Geometry check sheet. Reference: the model listing, model coordinates, mm. A direction names the side the tool comes from. Round coordinates to 2 decimals unless told otherwise and drop trailing zeros. Order: outer loops, then holes, each group sorted by start corner. A loop starts at its lowest first (then second) coordinate and runs counter-clockwise, first axis right, second up. Notation, with made-up numbers: M 81.25,-19 L 129.25,-19 A15 cw 129.25,-2 Z; hole C 65.5,6 d5. An arc over 180 degrees is marked long. Return JSON: item names as keys, results as strings. Group by question number.
```python
from build123d import *

# Parameters (mm, degrees)
F1_R     = 300
F1_R_2   = 275
F2_DEPTH = 25
F3_W     = 25
F3_H     = 25
F4_DEPTH = 410
F6_R     = 300
F6_R_2   = 275
F7_DEPTH = 25


with BuildPart() as f2:
    # F1 (on face) → F2 (new body)
    with BuildSketch(Plane.XY):
        Circle(F1_R)
        Circle(F1_R_2, mode=Mode.SUBTRACT)
    extrude(amount=F2_DEPTH)

    # F3 (on face) → F4 (join)
    with BuildSketch(Plane.XY.offset(25)):
        with Locations((0, 287.215762)):
            Rectangle(F3_W, F3_H)
        with Locations((-287.215762, 0)):
            Rectangle(F3_W, F3_H)
        with Locations((0, -287.215762)):
            Rectangle(F3_W, F3_H)
        with Locations((287.215762, 0)):
            Rectangle(F3_W, F3_H)
    extrude(amount=F4_DEPTH)

    # F6 (on offset) → F7 (join)
    with BuildSketch(Plane.XY.offset(435)):
        Circle(F6_R)
        Circle(F6_R_2, mode=Mode.SUBTRACT)
    extrude(amount=F7_DEPTH)


solid = f2.part
```
Q1. Depth check by flat-ended pin: pin 1 Ø7.5 at (y, z) = (-283.5, 160.5) entering from -X; pin 2 Ø20 at (x, z) = (-4, 245.5) entering from -Y; pin 3 Ø20 at (y, z) = (286.5, 318) entering from +X. Enter the tip coordinate at first touch or a pass-through.
Q2. Section check B-B on z = 268. Record the cut outline in (x, y), plus the area to 3 significant figures.
Q3. Release check for a two-part mould opening along X. For faces 1 (the face through (-39.054, 297.447, 447.325)), 2 (the face through (274.716, 0, 227)), 3 (the face through (132, -243, 435)) record: +X half, -X half, draft (parallel to the pull), parting line (faces both ways), or undercut.
Q4. Set-up check for faces 4 (the face through (287, 12.5, 227)), 5 (the face through (12.5, -287, 227)), 6 (the face through (0, -274.716, 227)), 7 (the face through (287, -12.5, 227)): record each of +Z, -Z, +X, -X, +Y, -Y from which the full face is reachable in a straight line by a thin tool's end or side.
Q5. Material ranges on line 1 along Z through (x, y) = (-217, -189.5); line 2 along Y through (x, z) = (-6.5, 208.5); line 3 along Y through (x, z) = (0, 443), recorded low to high.
Q6. Section check D-D on x = 200.5. Record the cut outline in (y, z), plus the area to 3 significant figures.
Q7. Section check A-A on x = 0. Record the cut outline in (y, z), plus the area to 3 significant figures.
Geometry check:
{
 "1": {"pin 1": "stops at x = -12.5", "pin 2": "stops at y = -299.72", "pin 3": "stops at x = 12.5"},
 "2": {"outline": "M -299.72,-12.5 L -274.72,-12.5 L -274.72,12.5 L -299.72,12.5 Z; M -12.5,-299.72 L 12.5,-299.72 L 12.5,-274.72 L -12.5,-274.72 Z; M -12.5,274.72 L 12.5,274.72 L 12.5,299.72 L -12.5,299.72 Z; M 274.72,-12.5 L 299.72,-12.5 L 299.72,12.5 L 274.72,12.5 Z", "area": "2,500 mm^2"},
 "3": {"face 1": "parting line", "face 2": "undercut", "face 3": "draft"},
 "4": {"face 4": "+X, -X, +Y", "face 5": "+X, +Y, -Y", "face 6": "+Z, -Z, +X, -X", "face 7": "+X, -X, -Y"},
 "5": {"line 1": "z = 0 to 25, 435 to 460", "line 2": "y = -299.72 to -274.72, 274.72 to 299.72", "line 3": "y = -300 to -275, 275 to 300"},
 "6": {"outline": "M -223.16,0 L -188.21,0 L -188.21,25 L -223.16,25 Z; M -223.16,435 L -188.21,435 L -188.21,460 L -223.16,460 Z; M 188.21,0 L 223.16,0 L 223.16,25 L 188.21,25 Z; M 188.21,435 L 223.16,435 L 223.16,460 L 188.21,460 Z", "area": "3,490 mm^2"},
 "7": {"outline": "M -300,0 L -275,0 L -275,25 L -274.72,25 L -274.72,435 L -275,435 L -275,460 L -300,460 L -300,435 L -299.72,435 L -299.72,25 L -300,25 Z; M 274.72,25 L 275,25 L 275,0 L 300,0 L 300,25 L 299.72,25 L 299.72,435 L 300,435 L 300,460 L 275,460 L 275,435 L 274.72,435 Z", "area": "23,000 mm^2"}
}
